Can you work these out from the model? Positions are in its coordinate system, mm. Round coordinates to 2 decimals unless told otherwise and drop trailing zeros. Loops run counter-clockwise (first coordinate to the right, second up) from the corner with the lowest first, then second, coordinate; pieces in that order, holes last.
(1) I want a section at A-A on y = 5.7. Give the number of separate pieces and of enclosed holes in the cut face, plus the area to 3 significant figures.
(2) I want a section at B-B on x = -82. Write out the boundary of the cut face in (y, z).
(3) Will this pin go through, and if not, where does the flat tip stop? pin 1 Ø1 at (y, z) = (6, -97) entering from +X.
(4) If I drill on line 1 along X through (y, z) = (5.7, 1.5); line 2 along X through (y, z) = (6.95, 72); line 3 along Z through (x, y) = (43, 6.7), over which ranges is the centre line in solid material (lowest first)?
Autodesk Inventor part; units mm, degrees
ref_plane "YZ Plane" through (0, 0, 0) normal (1, 0, 0) x (0, 1, 0)
ref_plane "XZ Plane" through (0, 0, 0) normal (0, 1, 0) x (-1, 0, 0)
ref_plane "XY Plane" through (0, 0, 0) normal (0, 0, 1) x (1, 0, 0)
ref_plane "Work Plane2" through (-4.4547, 5, 22.3935) normal (0, 1, 0) x (0.9711, 0, 0.2385)
sketch "Sketch2" plane through (-4.4547, 5, 22.3935) normal (0, 1, 0) x (0.9711, 0, 0.2385)
  line L0 (1.3055, 292.2458) -> (0.897, 292.9749)
  line L1 (165, 0) -> (82.5, 142.8942)
  line L2 (165, 0) -> (455.412, 0) construction
  line L3 (-165, 0) -> (-123.75, 71.4471)
  line L4 (-82.5, 142.8942) -> (82.5, 142.8942)
  line L5 (165, 0) -> (82.5384, -142.8363)
  line L6 (-165, 0) -> (-82.4975, -142.8985)
  line L7 (-82.4975, -142.8985) -> (82.5384, -142.8363)
  line L8 (-123.75, 71.4471) -> (123.7519, -71.4482)
  line L9 (-123.75, 71.4471) -> (-82.5, 142.8942)
  line L10 (-123.75, 71.4471) -> (-103.596, 106.3548)
  line L11 (-103.596, 106.3548) -> (-143.904, 36.5393)
  line L12 (-143.904, 36.5393) -> (-20.154, -34.9078)
  line L13 (-143.904, 36.5393) -> (-141.404, 40.8695)
  line L14 (-141.404, 40.8695) -> (-13.7235, -32.8469)
  line L15 (-143.904, 36.5393) -> (-140.154, 43.0345)
  line L16 (-140.154, 43.0345) -> (-8.7235, -32.8469)
  circle A0 centre (-122.1364, 29.7453) radius 1.25
  line L17 (-122.1364, 29.7453) -> (-104.8159, 19.7453)
  circle A1 centre (-104.8159, 19.7453) radius 1.25
  circle A2 centre (-119.6364, 34.0755) radius 1.25
  circle A3 centre (-102.3159, 24.0755) radius 1.25
  circle A4 centre (-86.8284, 90.9006) radius 1.25
  circle A5 centre (-69.5079, 80.9006) radius 1.25
  circle A6 centre (-72.0079, 76.5705) radius 1.25
  circle A7 centre (-89.3284, 86.5705) radius 1.25
  line L18 (-103.596, 106.3548) -> (38.9161, 24.0755)
  line L19 (0, -168.5342) -> (0, 201.2918)
  circle A8 centre (122.1364, 29.7453) radius 1.25
  circle A9 centre (104.8159, 19.7453) radius 1.25
  circle A10 centre (102.3159, 24.0755) radius 1.25
  circle A11 centre (119.6364, 34.0755) radius 1.25
  circle A12 centre (72.0079, 76.5705) radius 1.25
  circle A13 centre (89.3284, 86.5705) radius 1.25
  circle A14 centre (86.8284, 90.9006) radius 1.25
  circle A15 centre (69.5079, 80.9006) radius 1.25
  circle A16 centre (-35.308, -100.6459) radius 1.25
  circle A17 centre (30.308, -100.6459) radius 1.25
  circle A18 centre (35.308, -100.6459) radius 1.25
  circle A19 centre (30.308, -120.6459) radius 1.25
  circle A20 centre (35.308, -120.6459) radius 1.25
  circle A21 centre (-30.308, -100.6459) radius 1.25
  circle A22 centre (-30.308, -120.6459) radius 1.25
  circle A23 centre (-35.308, -120.6459) radius 1.25
  line L20 (-82.4975, -142.8985) -> (-65.177, -132.8985)
  line L21 (-82.4975, -142.8985) -> (-79.0334, -140.8985)
  line L22 (-165, 0) -> (-147.6795, 10)
  line L23 (-165, 0) -> (-145, 0) construction
  line L24 (-147.6795, 10) -> (-65.177, -132.8985)
  line L25 (-165, 0) -> (-161.5359, 2)
  line L26 (-161.5359, 2) -> (-79.0334, -140.8985)
  line L27 (-73.8372, -137.8985) -> (-156.3397, 5)
  line L28 (-79.0334, -140.8985) -> (-84.0334, -132.2383)
  line L29 (-84.0334, -132.2383) -> (-89.0334, -123.578)
  line L30 (-89.0334, -123.578) -> (-94.0334, -114.9178)
  line L31 (-123.7487, -71.4493) -> (-106.4282, -61.4493)
  circle A24 centre (-84.0334, -132.2383) radius 1.25
  circle A25 centre (-89.0334, -123.578) radius 1.25
  circle A26 centre (-94.0334, -114.9178) radius 1.25
  circle A27 centre (-73.6411, -126.2383) radius 1.25
  circle A28 centre (-78.6411, -117.578) radius 1.25
  circle A29 centre (-83.6411, -108.9178) radius 1.25
  circle A30 centre (-156.5359, -6.6603) radius 1.25
  circle A31 centre (-151.5359, -15.3205) radius 1.25
  circle A32 centre (-146.5359, -23.9808) radius 1.25
  circle A33 centre (-136.1436, -17.9808) radius 1.25
  circle A34 centre (-141.1436, -9.3205) radius 1.25
  circle A35 centre (-146.1436, -0.6603) radius 1.25
  circle A36 centre (72.505, 138.8942) radius 1.25
  circle A37 centre (62.505, 138.8942) radius 1.25
  circle A38 centre (52.505, 138.8942) radius 1.25
  circle A39 centre (52.505, 126.8942) radius 1.25
  circle A40 centre (62.505, 126.8942) radius 1.25
  circle A41 centre (72.505, 126.8942) radius 1.25
  circle A42 centre (-72.5, 138.8942) radius 1.25
  circle A43 centre (-62.5, 138.8942) radius 1.25
  circle A44 centre (-52.5, 138.8942) radius 1.25
  circle A45 centre (-52.5, 126.8942) radius 1.25
  circle A46 centre (-62.5, 126.8942) radius 1.25
  circle A47 centre (-72.5, 126.8942) radius 1.25
  circle A48 centre (84.0334, -132.2383) radius 1.25
  circle A49 centre (89.0334, -123.578) radius 1.25
  circle A50 centre (94.0334, -114.9178) radius 1.25
  circle A51 centre (83.6411, -108.9178) radius 1.25
  circle A52 centre (78.6411, -117.578) radius 1.25
  circle A53 centre (73.6411, -126.2383) radius 1.25
  circle A54 centre (156.5359, -6.6603) radius 1.25
  circle A55 centre (151.5359, -15.3205) radius 1.25
  circle A56 centre (146.5359, -23.9808) radius 1.25
  circle A57 centre (136.1436, -17.9808) radius 1.25
  circle A58 centre (141.1436, -9.3205) radius 1.25
  circle A59 centre (146.1436, -0.6603) radius 1.25
  dimension "d14" = 120
  dimension "d19" = 40.308
  dimension "d20" = 80.616
  dimension "d21" = 5
  dimension "d22" = 7.5
  dimension "d23" = 2.5
  dimension "d24" = 20
  dimension "d25" = 2.5
  dimension "d40" = 20
  dimension "d42" = 4
  dimension "d43" = 90
  dimension "d45" = 20
  dimension "d46" = 30
  dimension "d47" = 10
  dimension "d48" = 10
  dimension "d50" = 10
  dimension "d51" = 2.5
  dimension "d52" = 2.5
  dimension "d53" = 2.5
ref_plane "Work Plane3" through (-4.4547, 5, 22.3935) normal (0, 1, 0) x (0.9711, 0, 0.2385)
extrude "Extrusion2" add sketch "Sketch2" along normal blind 2 contours L5 L8 L19 L4 L1 | L5 L7 L19 L8 | L19 L18 L9 L4 | A1 L14 | L14 A1 | A0 L14 | L14 A0 | L19 L7 L20 L24 L22 L3 L8 | L8 L9 L18 L19 | L6 L31 L26 A26 A25 A24 L20 | L6 L22 L26 A30 A31 A32 L31 | L26 A24 A25 A26 L31 L27 L20 | L26 A32 A31 A30 L22 L27 L31 | L27 L31 L24 L20 | A24 L26 | L26 A24 | A32 L26 | L26 A32 | A26 L26 | L26 A26 | L27 L22 L24 L31 | A30 L26 | L26 A30 | A25 L26 | L26 A25 | A31 L26 | L26 A31 | A2 | A3 | A4 | A5 | A6 | A7 | A8 | A9 | A10 | A11 | A12 | A13 | A14 | A15 | A16 | A17 | A18 | A19 | A20 | A21 | A22 | A23 | A27 | A28 | A29 | A33 | A34 | A35 | A36 | A37 | A38 | A39 | A40 | A41 | A42 | A43 | A44 | A45 | A46 | A47 | A48 | A49 | A50 | A51 | A52 | A53 | A54 | A55 | A56 | A57 | A58 | A59
hole "Hole1" at (-98.0768, 5, -25.3881) at (-112.5127, 5, -39.2302) at (-115.9733, 5, -35.6213) at (-101.5374, 5, -21.7791) at (-70.56, 5, -82.9826) at (-67.0994, 5, -86.5915) at (-52.6635, 5, -72.7494) at (-56.1241, 5, -69.1404) direction (0, 1, 0) diameter 3 end through all
hole "Hole2" at (-67.5161, 5, 131.1379) at (-62.6604, 5, 132.3303) at (-62.7464, 5, 111.715) at (-57.8907, 5, 112.9074) at (-3.7934, 5, 146.7863) at (1.0623, 5, 147.9787) at (5.832, 5, 128.5558) at (0.9763, 5, 127.3634) at (102.0458, 5, 28.2148) at (100.6506, 5, 23.4134) at (121.2514, 5, 22.634) at (119.8562, 5, 17.8326) at (83.7364, 5, -34.7949) at (82.3412, 5, -39.5963) at (102.942, 5, -40.3757) at (101.5468, 5, -45.1771) direction (0, 1, 0) diameter 3 end through all
hole "Hole3" at (-44.6005, 5, -118.1295) at (-34.8891, 5, -115.7446) at (-25.1776, 5, -113.3598) at (-22.3158, 5, -125.0136) at (-32.0273, 5, -127.3984) at (-41.7387, 5, -129.7832) at (79.6595, 5, -99.9715) at (76.7976, 5, -88.3177) at (86.5091, 5, -85.9329) at (89.3709, 5, -97.5866) at (99.0824, 5, -95.2018) at (96.2206, 5, -83.548) at (-152.4816, 5, 10.7358) at (-140.9582, 5, 7.3873) at (-143.7486, 5, -2.2155) at (-155.2719, 5, 1.133) at (-158.0623, 5, -8.4698) at (-146.539, 5, -11.8183) at (-123.181, 5, 111.5699) at (-111.6576, 5, 108.2215) at (-108.8672, 5, 117.8243) at (-106.0769, 5, 127.4271) at (-117.6002, 5, 130.7755) at (-120.3906, 5, 121.1727) at (36.9557, 5, 162.5516) at (45.6172, 5, 170.8568) at (52.5383, 5, 163.6389) at (43.8767, 5, 155.3336) at (50.7978, 5, 148.1157) at (59.4593, 5, 156.4209) at (132.134, 5, 80.6288) at (123.4725, 5, 72.3235) at (130.3936, 5, 65.1056) at (139.0551, 5, 73.4109) at (145.9762, 5, 66.1929) at (137.3146, 5, 57.8876) direction (0, 1, 0) diameter 2.5 end through all
properties part number "ArmPlatform" material "Aluminum 6061"
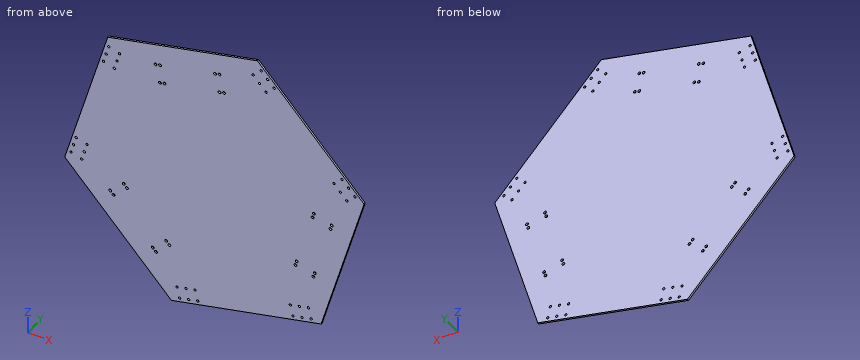
Filled sheet:
1. separate pieces: 1
1. enclosed holes: 60
1. area: 70,400 mm2
2. outline: (5, -103.2) - (7, -103.2) - (7, 150.48) - (5, 150.48) - close
3. pin 1: stops at x = 109.8
4. line 1: x = -159.33 to -156.47, -154.08 to 138.28
4. line 2: x = -138.85 to 122.27, 124.68 to 145.95
4. line 3: z = -113.09 to 154.44, 156.22 to 179.37
